Input: dimensioned drawing with shaded views. Units: mm. Origin: part minimum x, y, z. A direction names the side the tool comes from. Round coordinates to 2 decimals unless told otherwise and drop trailing zeros. Write each loop counter-clockwise with the first axis right and the second up, starting at its lowest first coordinate (ties: lowest second). Pieces come first, ordered by that corner, then holes. Notation, with made-up numbers: M -15.75,18.5 L 30.25,18.5 A23 ccw 30.25,54.5 Z; hole C 14,-3 d10. An arc over 180 degrees is marked long. Put each result on its own line as item: value. Start each with the question number.
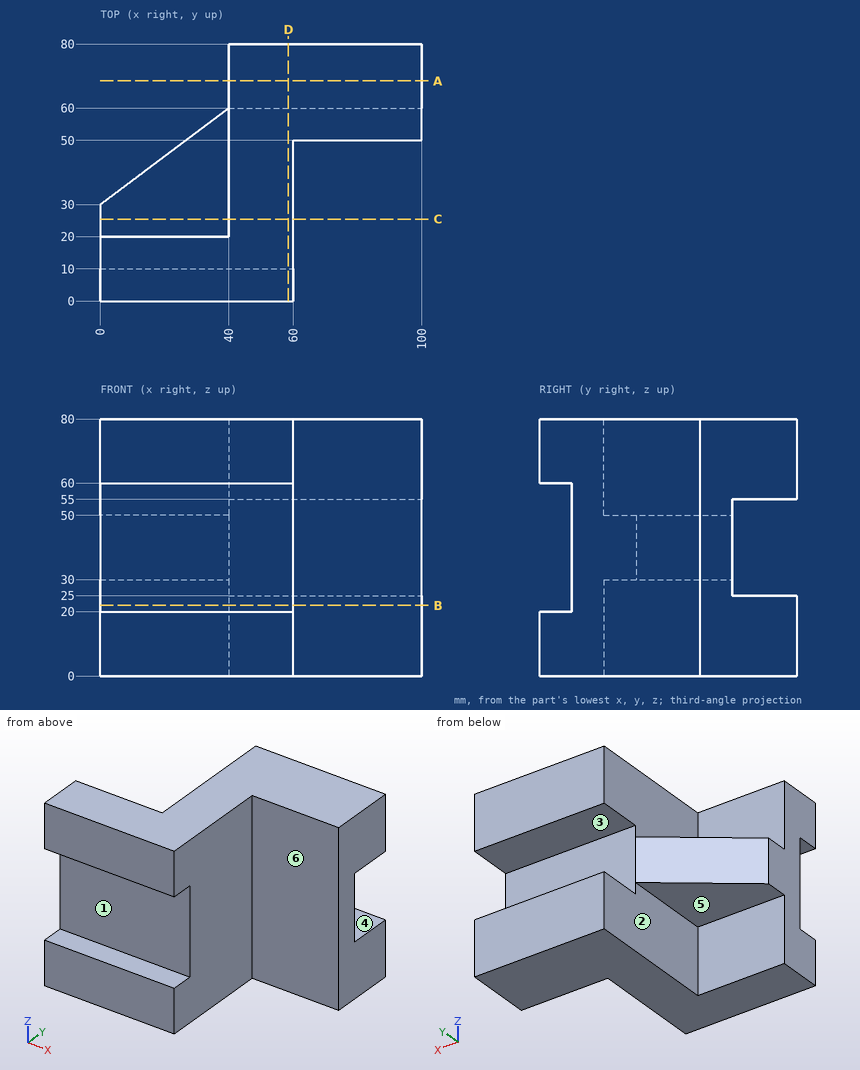
1) Section B-B, the plane z = 22. Output: boundary loops of the cut face in (x, y), and give its area (3 significant figures).
2) Ray query, probe 1 along Z at (x, y) = (47, 72); probe 2 along Z at (x, y) = (26.5, 3); probe 3 along Y at (x, z) = (36, 19.5). Return the intervals inside material, ascending.
3) Draft query along Z for the marked faces 4, 5 and 6. Return one class per face: +Z half, -Z half, draft (parallel to the pull), parting line (faces both ways), or undercut.
4) Section A-A, the plane y = 68.5. Output: boundary loops of the cut face in (x, z).
5) Section C-C, the plane y = 25.5. Output: boundary loops of the cut face in (x, z).
6) First-contact query: pin 1 (20 mm diameter, centred on x = 28, y = 46, fed in from -Z); pin 2 (5 mm diameter, centred on y = 43, z = 16.5, fed in from -X); pin 3 (8 mm diameter, centred on y = 38.5, z = 32, fed in from +X). Flat tips, straight axial feed; report the tip coordinate or a pass-through.
7) Access query for the marked faces 1, 2 and 3. Directions: +Z, -Z, +X, -X, +Y, -Y. A direction counts if a zero-diameter tool reaches every point of the face in a straight line with its end or side. Return the directions, or none.
8) Section D-D, the plane x = 58.5. Output: boundary loops of the cut face in (y, z), and give its area (3 significant figures).
Solved:
1. outline: M 0,10 L 60,10 L 60,50 L 100,50 L 100,80 L 40,80 L 40,20 L 0,20 Z
1. area: 3,000 mm2
2. probe 1: z = 0 to 25, 55 to 80
2. probe 2: z = 0 to 20, 60 to 80
2. probe 3: y = 0 to 20
3. face 4: undercut
3. face 5: -Z half
3. face 6: draft
4. outline: M 40,0 L 100,0 L 100,25 L 40,25 Z; M 40,55 L 100,55 L 100,80 L 40,80 Z
5. outline: M 0,30 L 40,30 L 40,0 L 60,0 L 60,80 L 40,80 L 40,50 L 0,50 Z
6. pin 1: stops at z = 30
6. pin 2: stops at x = 40
6. pin 3: stops at x = 60
7. face 1: +X, -X, -Y
7. face 2: -Z, -X, +Y
7. face 3: +X, -X, +Y
8. outline: M 0,0 L 80,0 L 80,25 L 60,25 L 60,55 L 80,55 L 80,80 L 0,80 L 0,60 L 10,60 L 10,20 L 0,20 Z
8. area: 5,400 mm2
